Input: part model. Units: mm. Frame: model coordinates. Face numbers are marked on the shaded views. A direction names the side the tool comes from. Round coordinates to 2 decimals unless told otherwise and drop trailing zeros. Loops run counter-clockwise (first coordinate to the right, second up) from the corner with the lowest first, then second, coordinate; pieces in that order, holes last. Notation, with made-up numbers: M 15.5,16 L 65.5,16 A9 cw 65.5,27 Z; hole C 57.5,82.5 d5. An arc over 180 degrees is marked long. Use one line per item in the form item = value. Start each with the question number.
Q1. Section query B-B, the plane y = 0. Output: boundary loops of the cut face in (x, z).
Q2. First-contact query: P1, Ø10, axis at x = 5.5, z = 3, coming from the -Y side; P2, Ø1.5, axis at x = -1.5, z = 1, coming from the +Y side. Flat tips, straight axial feed; report the tip coordinate or a pass-through.
Q3. Access query for the marked faces 1 and 2. Directions: +Z, -Z, +X, -X, +Y, -Y. A direction counts if a zero-diameter tool reaches every point of the face in a straight line with its end or side. Return the directions, or none.
Q4. Mould query, pull axis Z, two halves, no side actions, for the marked faces 3, 4, 5 and 6. Classes: pulls with the +Z half, pulls with the -Z half, needs draft (parallel to the pull), parting line crosses it, or undercut.
Q5. Section query D-D, the plane z = -5. Output: boundary loops of the cut face in (x, y).
Q6. Ray query, line 1 along Y through (x, z) = (6.5, -7.75); line 2 along Y through (x, z) = (6.5, -1.5); line 3 along Z through (x, y) = (-0.75, 4.25). Return the intervals inside material, ascending.
Q7. Section query A-A, the plane x = 6.5. Output: boundary loops of the cut face in (y, z), and give its area (3 significant figures).
Q8. Section query C-C, the plane z = -1.5. Output: boundary loops of the cut face in (x, y), and give its area (3 significant figures).
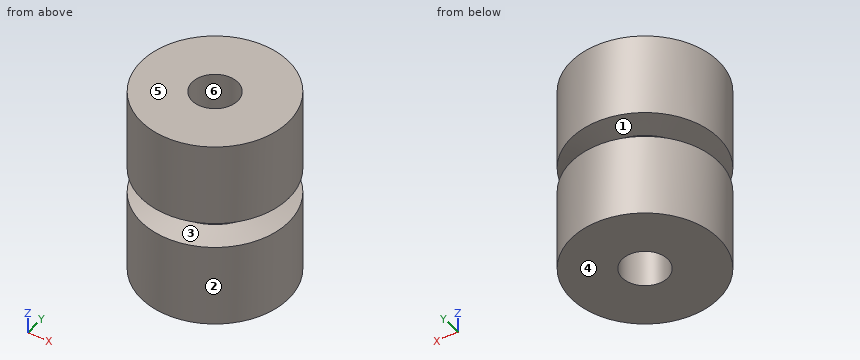
Autodesk Inventor part; units mm, degrees
ref_plane "YZ Plane" through (0, 0, 0) normal (1, 0, 0) x (0, 1, 0)
ref_plane "XZ Plane" through (0, 0, 0) normal (0, 1, 0) x (-1, 0, 0)
ref_plane "XY Plane" through (0, 0, 0) normal (0, 0, 1) x (1, 0, 0)
sketch "Sketch1" plane through (0, 0, 0) normal (0, 1, 0) x (-1, 0, 0)
  line L0 (0, 0) -> (0, -2.5)
  line L1 (3.5, 0.5) -> (0, 0)
  line L2 (3.5, -3) -> (0, -2.5)
  line L3 (3.5, -3) -> (3.5, -14.25)
  line L4 (3.5, -14.25) -> (-6.5, -14.25)
  line L5 (3.5, 0.5) -> (3.5, 11.75)
  line L6 (3.5, 11.75) -> (-6.5, 11.75)
  line L7 (-6.5, 11.75) -> (-6.5, -14.25)
  dimension "d0" = 2.5
  dimension "d6" = 3.5
  dimension "d9" = 11.25
  dimension "d11" = 10
  dimension "d12" = 90
  dimension "d13" = 11.25
  dimension "d15" = 10
  dimension "d16" = 90
  dimension "d17" = 3.5
  dimension "d18" = 11.75
revolve "Revolution1" add sketch "Sketch1" angle 360 about axis through (6.5, 0, 11.75) along (0, 0, -1)
sketch "Sketch2" plane through (6.5, 0, -14.25) normal (0, 0, -1) x (-1, 0, 0)
  circle A0 centre (0, 0) radius 3.1
  circle A1 centre (0, 0) radius 10
  point P0 (6.5, 0)
  dimension "d20" = 6.2
extrude "Extrusion1" cut sketch "Sketch2" against normal blind 26 contours A0
properties part number "roller" material "ABS Plastic"
Results found:
q1.outline = M -3.5,-14.25 L 3.4,-14.25 L 3.4,11.75 L -3.5,11.75 L -3.5,0.5 L 0,0 L 0,-2.5 L -3.5,-3 Z; M 9.6,-14.25 L 16.5,-14.25 L 16.5,-3 L 13,-2.5 L 13,0 L 16.5,0.5 L 16.5,11.75 L 9.6,11.75 Z
q2.P1 = -10
q2.P2 = 6.89
q3.face_1 = none
q3.face_2 = +Z, -Z
q4.face_3 = undercut
q4.face_4 = pulls with the -Z half
q4.face_5 = pulls with the +Z half
q4.face_6 = needs draft
q5.outline = C 6.5,0 d20; hole C 6.5,0 d6.2
q6.line_1 = -10 to -3.1, 3.1 to 10
q6.line_2 = -6.5 to -3.1, 3.1 to 6.5
q6.line_3 = -14.25 to -2.77, 0.27 to 11.75
q7.outline = M -10,-14.25 L -3.1,-14.25 L -3.1,11.75 L -10,11.75 L -10,0.5 L -6.5,0 L -6.5,-2.5 L -10,-3 Z; M 3.1,-14.25 L 10,-14.25 L 10,-3 L 6.5,-2.5 L 6.5,0 L 10,0.5 L 10,11.75 L 3.1,11.75 Z
q7.area = 338 mm²
q8.outline = C 6.5,0 d13; hole C 6.5,0 d6.2
q8.area = 103 mm²
